Work out the finished part from the listing and answer in its coordinate system (mm). Give positions to 0.01 mm unless a question says otherwise; leave off trailing zeros. Loops run counter-clockwise (first coordinate to the right, second up) from the corner with the lowest first, then second, coordinate; pieces in that order, holes last. Notation, with made-up numbers: M 18.5,-21.75 L 33.5,-21.75 A28 cw 33.5,4.25 Z; hole C 49.25,20.5 d1. An arc over 180 degrees is marked long. Write item = value, one per line. Start each with the question number.
1. Section B-B on z = -18.75 is taken. Determine the outline of the cut face in (x, y).
2. Flat-ended cylindrical pins translate along their axes: pin 1 Ø6.5 at (y, z) = (-55, -40) entering from +X; pin 2 Ø3.5 at (y, z) = (-47.33, 40) entering from -X. Find the tip coordinate at first contact, or state that the pin passes through.
3. The mould has two halves that part along Z. Classify faces 1 (the face through (3, -65, 2)), 2 (the face through (2.88, -56.01, -77.57)): released by +Z, released by -Z, zero draft, split by the parting line, or undercut.
4. Consider L1, parallel to Y at x = 0.85, z = 0; L2, parallel to Z at x = 1.35, y = 55; L3, parallel to Y at x = 5.05, z = 36. Determine where each line is inside the solid, lowest interval first. Write a range as [from, to].
5. Section A-A on y = 55 is taken. Give the number of separate pieces and of enclosed holes in the cut face, plus the area to 3 significant figures.
```python
from build123d import *

# Parameters (mm, degrees)
SKETCH1_W                                            = 227.5
SKETCH1_H                                            = 130
BOSS_EXTRUDE1_DEPTH                                  = 5.5
CSK_FOR_M5_HEX_SOCKET_COUNTERSUNK_CAP_SC_D           = 5
CSK_FOR_M5_HEX_SOCKET_COUNTERSUNK_CAP_SC_CSINK_D     = 10.5
CSK_FOR_M5_HEX_SOCKET_COUNTERSUNK_CAP_SC_CSINK_ANGLE = 90
TAP_DRILL_FOR_M5X0_8_TAP1_D                          = 5
SKETCH9_R                                            = 1.5
CUT_EXTRUDE1_DEPTH                                   = 29
SKETCH10_R                                           = 1.5
CUT_EXTRUDE2_DEPTH                                   = 29


with BuildPart() as part:
    # Sketch1 → Boss-Extrude1 (new body)
    with BuildSketch(Plane(origin=(0, 0, 0), x_dir=(0, 0, -1), z_dir=(1, 0, 0))):
        Rectangle(SKETCH1_W, SKETCH1_H)
    extrude(amount=BOSS_EXTRUDE1_DEPTH)

    # CSK for M5 Hex Socket Countersunk Cap Screw1 (through all)
    with Locations(Plane(origin=(5.5, 0, 0), x_dir=(0, 0, -1), z_dir=(1, 0, 0))):
        with Locations((80, 55), (40, 55), (0, 55), (-40, 55), (-80, 55), (-80, -55), (-40, -55), (0, -55), (40, -55), (80, -55)):
            CounterSinkHole(CSK_FOR_M5_HEX_SOCKET_COUNTERSUNK_CAP_SC_D / 2, CSK_FOR_M5_HEX_SOCKET_COUNTERSUNK_CAP_SC_CSINK_D / 2, counter_sink_angle=CSK_FOR_M5_HEX_SOCKET_COUNTERSUNK_CAP_SC_CSINK_ANGLE)

    # Tap Drill for M5x0.8 Tap1 (through all)
    with Locations(Plane(origin=(5.5, 0, 0), x_dir=(0, 0, -1), z_dir=(1, 0, 0))):
        with Locations((-63.75, -52.653836842), (-18.75, -52.653836842), (18.75, -52.653836842), (63.75, -52.653836842)):
            Hole(TAP_DRILL_FOR_M5X0_8_TAP1_D / 2)

    # Sketch9 → Cut-Extrude1 (cut)
    with BuildSketch(Plane.ZY):
        with Locations((-80.045792536, -47.3325)):
            Circle(SKETCH9_R)
        with Locations((-40, -47.3325)):
            Circle(SKETCH9_R)
        with Locations((0, -47.3325)):
            Circle(SKETCH9_R)
        with Locations((40, -47.3325)):
            Circle(SKETCH9_R)
        with Locations((80, -47.3325)):
            Circle(SKETCH9_R)
    extrude(amount=-CUT_EXTRUDE1_DEPTH, mode=Mode.SUBTRACT)

    # Sketch10 → Cut-Extrude2 (cut)
    with BuildSketch(Plane.ZY):
        with Locations((-80, 47.3325)):
            Circle(SKETCH10_R)
        with Locations((-40, 47.3325)):
            Circle(SKETCH10_R)
        with Locations((0, 47.3325)):
            Circle(SKETCH10_R)
        with Locations((40, 47.3325)):
            Circle(SKETCH10_R)
        with Locations((80, 47.3325)):
            Circle(SKETCH10_R)
    extrude(amount=-CUT_EXTRUDE2_DEPTH, mode=Mode.SUBTRACT)


solid = part.part
```
Verdict:
q1.outline = M 0,-65 L 5.5,-65 L 5.5,-55.15 L 0,-55.15 Z; M 0,-50.15 L 5.5,-50.15 L 5.5,65 L 0,65 Z
q2.pin_1 = 3.5
q2.pin_2 = 0
q3.face_1 = zero draft
q3.face_2 = undercut
q4.L1 = [-65, -57.5], [-52.5, -48.83], [-45.83, 45.83], [48.83, 52.5], [57.5, 65]
q4.L2 = [-113.75, -82.5], [-77.5, -42.5], [-37.5, -2.5], [2.5, 37.5], [42.5, 77.5], [82.5, 113.75]
q4.L3 = [-65, -57.65], [-52.35, 52.35], [57.65, 65]
q5.separate_pieces = 6
q5.enclosed_holes = 0
q5.area = 1,080 mm2
